Verification items for the finished model (mm, model axes). Give positions to 0.01 mm unless a question says otherwise; leave off trailing zeros. Loops run counter-clockwise (first coordinate to the right, second up) from the corner with the lowest first, then second, coordinate; pieces in that order, holes last. Notation, with made-up numbers: (12, 50.5) - (50, 50.5) arc R28 ccw to (50, 69.5) - close; hole circle Ø11 at (84, -29.75). An arc over 180 degrees is marked (long way). Put each result on its own line as item: value. Start each with the question number.
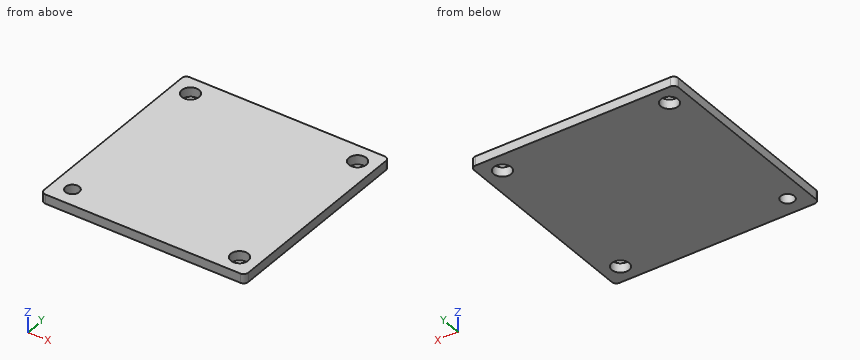
```python
from build123d import *

# Parameters (mm, degrees)
F0_W     = 139.7
F0_H     = 139.7
F0_R     = 5.953125
F1_DEPTH = 6.35
F3_D     = 9.3472
F4_R     = 3.175
F5_R     = 3.175
F6_R     = 3.175
F7_R     = 3.175


with BuildPart() as f1:
    # F0 (on Top) → F1 (new body)
    with BuildSketch(Plane.XY):
        Rectangle(F0_W, F0_H)
        with Locations((-57.15, -57.15)):
            Circle(F0_R, mode=Mode.SUBTRACT)
        with Locations((57.15, -57.15)):
            Circle(F0_R, mode=Mode.SUBTRACT)
        with Locations((-57.15, 57.15)):
            Circle(F0_R, mode=Mode.SUBTRACT)
        with Locations((57.15, 57.15)):
            Circle(F0_R, mode=Mode.SUBTRACT)
        with Locations((-57.15, -57.15)):
            Circle(F0_R)
    extrude(amount=F1_DEPTH)

    # F3 (through all)
    with Locations(Plane.XY.offset(6.35)):
        with Locations((-57.15, -57.15)):
            Hole(F3_D / 2)

    # F4
    f4_edges = [f1.edges().sort_by_distance(p)[0] for p in [
        (-69.85, 69.85, 3.175),
    ]]
    fillet(f4_edges, radius=F4_R)

    # F5
    f5_edges = [f1.edges().sort_by_distance(p)[0] for p in [
        (69.85, 69.85, 3.175),
    ]]
    fillet(f5_edges, radius=F5_R)

    # F6
    f6_edges = [f1.edges().sort_by_distance(p)[0] for p in [
        (69.85, -69.85, 3.175),
    ]]
    fillet(f6_edges, radius=F6_R)

    # F7
    f7_edges = [f1.edges().sort_by_distance(p)[0] for p in [
        (-69.85, -69.85, 3.175),
    ]]
    fillet(f7_edges, radius=F7_R)


solid = f1.part
```
1) Section check B-B, the plane x = -57.15. Enter the section's corners in (y, z).
2) Scan lines: line 1 along Y through (x, z) = (-57.15, 3.75); line 2 along Y through (x, z) = (57.15, 3); line 3 along X through (y, z) = (-55, 4.5). Record each from-to range of solid material in increasing order. Write a range as from..to.
3) Section check C-C, the plane z = 5. Enter the section's corners in (x, y) (3 decimals).
4) Depth check by flat-ended pin: P1, Ø7, axis at x = 57.15, y = 57.15, coming from the +Z side. Enter the tip coordinate at first touch or a pass-through.
5) Section check A-A, the plane y = 57.15. Enter the section's corners in (x, z), plus the area to 3 significant figures.
Results are:
1. outline: (-69.85, 0) - (-61.82, 0) - (-61.82, 6.35) - (-69.85, 6.35) - close; (-52.48, 0) - (51.2, 0) - (51.2, 6.35) - (-52.48, 6.35) - close; (63.1, 0) - (69.85, 0) - (69.85, 6.35) - (63.1, 6.35) - close
2. line 1: y = -69.85..-61.82, -52.48..51.2, 63.1..69.85
2. line 2: y = -69.85..-63.1, -51.2..51.2, 63.1..69.85
2. line 3: x = -69.85..-61.3, -53..51.6, 62.7..69.85
3. outline: (-69.85, -66.675) arc R3.175 ccw to (-66.675, -69.85) - (66.675, -69.85) arc R3.175 ccw to (69.85, -66.675) - (69.85, 66.675) arc R3.175 ccw to (66.675, 69.85) - (-66.675, 69.85) arc R3.175 ccw to (-69.85, 66.675) - close; hole circle Ø11.906 at (-57.15, 57.15); hole circle Ø9.347 at (-57.15, -57.15); hole circle Ø11.906 at (57.15, -57.15); hole circle Ø11.906 at (57.15, 57.15)
4. P1: passes through
5. outline: (-69.85, 0) - (-63.1, 0) - (-63.1, 6.35) - (-69.85, 6.35) - close; (-51.2, 0) - (51.2, 0) - (51.2, 6.35) - (-51.2, 6.35) - close; (63.1, 0) - (69.85, 0) - (69.85, 6.35) - (63.1, 6.35) - close
5. area: 736 mm2
